from build123d import *

# Parameters (mm, degrees)
SKETCH1_W           = 400
SKETCH1_H           = 200
SKETCH1_W_2         = 8.5
SKETCH1_H_2         = 8.5
BOSS_EXTRUDE1_DEPTH = 10
FILLET2_R           = 2
CUT_EXTRUDE1_REACH  = 225.83
SKETCH2_R           = 2.375
FILLET3_R           = 10
SKETCH3_R           = 3.4
CUT_EXTRUDE3_DEPTH  = 20


with BuildPart() as part:
    # Sketch1 → Boss-Extrude1 (new body)
    # profile 1 of 9: a face of its own
    with BuildSketch(Plane.XY):
        Rectangle(SKETCH1_W, SKETCH1_H)
        Polygon((-128.55, 28.25), (-120.05, 28.25), (-80.55, 28.25), (-72.05, 28.25), (-72.05, 19.75), (-72.05, -19.75), (-72.05, -28.25), (-80.55, -28.25), (-120.05, -28.25), (-128.55, -28.25), (-128.55, -19.75), (-128.55, 19.75), align=None, mode=Mode.SUBTRACT)
        Polygon((51.75, 19.75), (51.75, 28.25), (60.25, 28.25), (99.75, 28.25), (108.25, 28.25), (108.25, 19.75), (108.25, -19.75), (108.25, -28.25), (99.75, -28.25), (60.25, -28.25), (51.75, -28.25), (51.75, -19.75), align=None, mode=Mode.SUBTRACT)
    # profile 2 of 9: a face of its own
    with BuildSketch(Plane.XY):
        with Locations((-124.3, 24)):
            Rectangle(SKETCH1_W_2, SKETCH1_H_2)
    # profile 3 of 9: a face of its own
    with BuildSketch(Plane.XY):
        with Locations((-76.3, 24)):
            Rectangle(SKETCH1_W_2, SKETCH1_H_2)
    # profile 4 of 9: a face of its own
    with BuildSketch(Plane.XY):
        with Locations((-76.3, -24)):
            Rectangle(SKETCH1_W_2, SKETCH1_H_2)
    # profile 5 of 9: a face of its own
    with BuildSketch(Plane.XY):
        with Locations((-124.3, -24)):
            Rectangle(SKETCH1_W_2, SKETCH1_H_2)
    # profile 6 of 9: a face of its own
    with BuildSketch(Plane.XY):
        with Locations((56, -24)):
            Rectangle(SKETCH1_W_2, SKETCH1_H_2)
    # profile 7 of 9: a face of its own
    with BuildSketch(Plane.XY):
        with Locations((56, 24)):
            Rectangle(SKETCH1_W_2, SKETCH1_H_2)
    # profile 8 of 9: a face of its own
    with BuildSketch(Plane.XY):
        with Locations((104, 24)):
            Rectangle(SKETCH1_W_2, SKETCH1_H_2)
    # profile 9 of 9: a face of its own
    with BuildSketch(Plane.XY):
        with Locations((104, -24)):
            Rectangle(SKETCH1_W_2, SKETCH1_H_2)
    extrude(amount=BOSS_EXTRUDE1_DEPTH)

    # Fillet2
    fillet2_edges = [part.edges().sort_by_distance(p)[0] for p in [
        (60.25, 19.75, 5),
        (60.25, -19.75, 5),
        (99.75, -19.75, 5),
        (99.75, 19.75, 5),
        (-80.55, 19.75, 5),
        (-120.05, 19.75, 5),
        (-120.05, -19.75, 5),
        (-80.55, -19.75, 5),
    ]]
    fillet(fillet2_edges, radius=FILLET2_R)

    # Sketch2 → Cut-Extrude1 (cut, up to next)
    with BuildSketch(Plane(origin=(0, 0, 0), x_dir=(-1, 0, 0), z_dir=(0, 0, -1)), mode=Mode.PRIVATE) as cut_extrude1_sk1:
        with Locations((-103.57, 23.57)):
            Circle(SKETCH2_R)
    cut_extrude1_tool1 = extrude(cut_extrude1_sk1.sketch, amount=-CUT_EXTRUDE1_REACH, mode=Mode.PRIVATE) & part.part
    # Sketch2 → Cut-Extrude1 (cut, up to next)
    with BuildSketch(Plane(origin=(0, 0, 0), x_dir=(-1, 0, 0), z_dir=(0, 0, -1)), mode=Mode.PRIVATE) as cut_extrude1_sk2:
        with Locations((-56.43, 23.57)):
            Circle(SKETCH2_R)
    cut_extrude1_tool2 = extrude(cut_extrude1_sk2.sketch, amount=-CUT_EXTRUDE1_REACH, mode=Mode.PRIVATE) & part.part
    # Sketch2 → Cut-Extrude1 (cut, up to next)
    with BuildSketch(Plane(origin=(0, 0, 0), x_dir=(-1, 0, 0), z_dir=(0, 0, -1)), mode=Mode.PRIVATE) as cut_extrude1_sk3:
        with Locations((-56.43, -23.57)):
            Circle(SKETCH2_R)
    cut_extrude1_tool3 = extrude(cut_extrude1_sk3.sketch, amount=-CUT_EXTRUDE1_REACH, mode=Mode.PRIVATE) & part.part
    # Sketch2 → Cut-Extrude1 (cut, up to next)
    with BuildSketch(Plane(origin=(0, 0, 0), x_dir=(-1, 0, 0), z_dir=(0, 0, -1)), mode=Mode.PRIVATE) as cut_extrude1_sk4:
        with Locations((-103.57, -23.57)):
            Circle(SKETCH2_R)
    cut_extrude1_tool4 = extrude(cut_extrude1_sk4.sketch, amount=-CUT_EXTRUDE1_REACH, mode=Mode.PRIVATE) & part.part
    # Sketch2 → Cut-Extrude1 (cut, up to next)
    with BuildSketch(Plane(origin=(0, 0, 0), x_dir=(-1, 0, 0), z_dir=(0, 0, -1)), mode=Mode.PRIVATE) as cut_extrude1_sk5:
        with Locations(Location((123.87, -23.57, 0), (0, 0, 180))):
            Circle(SKETCH2_R)
    cut_extrude1_tool5 = extrude(cut_extrude1_sk5.sketch, amount=-CUT_EXTRUDE1_REACH, mode=Mode.PRIVATE) & part.part
    # Sketch2 → Cut-Extrude1 (cut, up to next)
    with BuildSketch(Plane(origin=(0, 0, 0), x_dir=(-1, 0, 0), z_dir=(0, 0, -1)), mode=Mode.PRIVATE) as cut_extrude1_sk6:
        with Locations(Location((76.73, -23.57, 0), (0, 0, 180))):
            Circle(SKETCH2_R)
    cut_extrude1_tool6 = extrude(cut_extrude1_sk6.sketch, amount=-CUT_EXTRUDE1_REACH, mode=Mode.PRIVATE) & part.part
    # Sketch2 → Cut-Extrude1 (cut, up to next)
    with BuildSketch(Plane(origin=(0, 0, 0), x_dir=(-1, 0, 0), z_dir=(0, 0, -1)), mode=Mode.PRIVATE) as cut_extrude1_sk7:
        with Locations(Location((76.73, 23.57, 0), (0, 0, 180))):
            Circle(SKETCH2_R)
    cut_extrude1_tool7 = extrude(cut_extrude1_sk7.sketch, amount=-CUT_EXTRUDE1_REACH, mode=Mode.PRIVATE) & part.part
    # Sketch2 → Cut-Extrude1 (cut, up to next)
    with BuildSketch(Plane(origin=(0, 0, 0), x_dir=(-1, 0, 0), z_dir=(0, 0, -1)), mode=Mode.PRIVATE) as cut_extrude1_sk8:
        with Locations(Location((123.87, 23.57, 0), (0, 0, 180))):
            Circle(SKETCH2_R)
    cut_extrude1_tool8 = extrude(cut_extrude1_sk8.sketch, amount=-CUT_EXTRUDE1_REACH, mode=Mode.PRIVATE) & part.part
    add(cut_extrude1_tool1.solids().sort_by_distance((103.57, 23.57, 0))[0], mode=Mode.SUBTRACT)
    add(cut_extrude1_tool2.solids().sort_by_distance((56.43, 23.57, 0))[0], mode=Mode.SUBTRACT)
    add(cut_extrude1_tool3.solids().sort_by_distance((56.43, -23.57, 0))[0], mode=Mode.SUBTRACT)
    add(cut_extrude1_tool4.solids().sort_by_distance((103.57, -23.57, 0))[0], mode=Mode.SUBTRACT)
    add(cut_extrude1_tool5.solids().sort_by_distance((-123.87, -23.57, 0))[0], mode=Mode.SUBTRACT)
    add(cut_extrude1_tool6.solids().sort_by_distance((-76.73, -23.57, 0))[0], mode=Mode.SUBTRACT)
    add(cut_extrude1_tool7.solids().sort_by_distance((-76.73, 23.57, 0))[0], mode=Mode.SUBTRACT)
    add(cut_extrude1_tool8.solids().sort_by_distance((-123.87, 23.57, 0))[0], mode=Mode.SUBTRACT)

    # Fillet3
    fillet3_edges = [part.edges().sort_by_distance(p)[0] for p in [
        (-200, 100, 5),
        (200, 100, 5),
        (200, -100, 5),
        (-200, -100, 5),
    ]]
    fillet(fillet3_edges, radius=FILLET3_R)

    # Sketch3 → Cut-Extrude3 (cut)
    with BuildSketch(Plane(origin=(0, 0, 0), x_dir=(-1, 0, 0), z_dir=(0, 0, -1))):
        with Locations((84.3, -52.25)):
            Circle(SKETCH3_R)
        with Locations((116.3, -52.25)):
            Circle(SKETCH3_R)
        with Locations((84.3, 52.25)):
            Circle(SKETCH3_R)
        with Locations((116.3, 52.25)):
            Circle(SKETCH3_R)
    extrude(amount=-CUT_EXTRUDE3_DEPTH, mode=Mode.SUBTRACT)


solid = part.part
Can you work these out from the model? Positions are in its coordinate system, mm. A direction names the side the tool comes from. Coordinates: 2 decimals unless noted, no trailing zeros. Loops run counter-clockwise (first coordinate to the right, second up) from the corner with the lowest first, then second, coordinate; pieces in that order, holes last. Notation, with made-up numbers: (8, 85) - (20, 85) arc R22 ccw to (20, 114) - close; hole circle Ø3 at (23, -1.75). An arc over 180 degrees is marked (long way). Answer as a JSON object with one key per item and string values. Group by question number.
Item 1: If we section it at A-A (y = 11): List the corners of the cut face in (x, z) for me.
Item 2: On a 3-axis mill with a long thin cutter (end or side, diameter ignored), from which of +Z, -Z, +X, -X, +Y, -Y can I reach the whole of each face in a straight line? I mean faces 5 (the face through (80, -28.25, 5)), 6 (the face through (-3, 1, 10)). Say none if no direction works.
Item 3: If we section it at C-C (z = 3.25): State how many separate pieces and enclosed holes the cut face has, plus the area to 3 significant figures.
Item 4: If we section it at B-B (x = 94): List the corners of the cut face in (y, z) for me, plus the area to 4 significant figures.
Item 5: If we mould it in two halves opening along X, with no side actions, what happens to faces 1 (the face through (-3, 100, 5)), 2 (the face through (196.99, -97.15, 5.07)), 3 (the face through (80, 28.25, 5)), 4 (the face through (-197.15, 96.99, 5.07))? For each: released by +X, released by -X, zero draft, split by the parting line, or undercut.
Item 6: If I drill on L1, parallel to Y at x = -117, z = 5.75; L2, parallel to Y at x = -123.87, z = 6.75 (3 decimals); L3, parallel to X at y = 16.5, z = 4.25, over which ranges is the centre line in solid material (lowest first)? Write a range as from..to.
Returned:
{
 "1": {"outline": "(-200, 0) - (-128.55, 0) - (-128.55, 10) - (-200, 10) - close; (-72.05, 0) - (51.75, 0) - (51.75, 10) - (-72.05, 10) - close; (108.25, 0) - (200, 0) - (200, 10) - (108.25, 10) - close"},
 "2": {"face 5": "+Z, -Z", "face 6": "+Z, +X, -X, +Y, -Y"},
 "3": {"separate pieces": "1", "enclosed holes": "14", "area": "73,800 mm²"},
 "4": {"outline": "(-100, 0) - (-28.25, 0) - (-28.25, 10) - (-100, 10) - close; (28.25, 0) - (100, 0) - (100, 10) - (28.25, 10) - close", "area": "1,435 mm²"},
 "5": {"face 1": "zero draft", "face 2": "released by +X", "face 3": "undercut", "face 4": "released by -X"},
 "6": {"L1": "y = -100..-55.58, -48.92..-28.25, 28.25..48.92, 55.58..100", "L2": "y = -100..-25.945, -21.195..-19.75, 19.75..21.195, 25.945..100", "L3": "x = -200..-128.55, -72.05..51.75, 108.25..200"}
}
